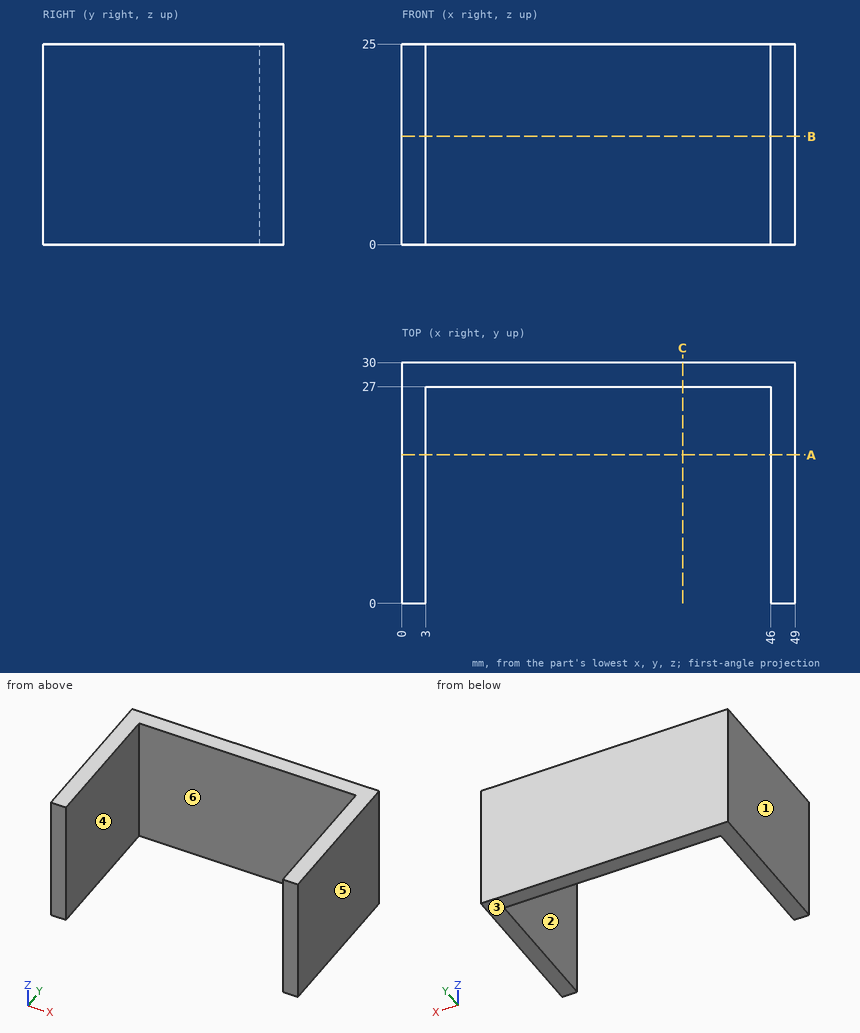
Geometry: see drawing. Coordinates: mm, zero at the bounding-box minimum. A direction names the side the tool comes from. Coordinates: 2 decimals unless noted, no trailing zeros. Loops run counter-clockwise (first coordinate to the right, second up) from the corner with the lowest first, then second, coordinate; pieces in that order, holes last. Notation, with made-up numbers: (18, 14.5) - (47, 14.5) arc R15 cw to (47, 35.5) - close; hole circle Ø10 at (27.25, 26.5). An arc over 180 degrees is marked (long way). Answer in a Markdown table with one row per item.
(1) Set-up query: the marked faces 5 and 6. Return all of +Z, -Z, +X, -X, +Y, -Y with unobstructed straight access to the full face (end or side cutting, diameter ignored); none if empty.
Model answer:
| item | result |
|---|---|
| face 5 | +Z, -Z, +X, +Y, -Y |
| face 6 | +Z, -Z, -Y |
(2) Cut plane C-C on x = 35. Output: boundary loops of the cut face in (y, z), plus the area to 3 significant figures.
Model answer:
| item | result |
|---|---|
| outline | (27, 0) - (30, 0) - (30, 25) - (27, 25) - close |
| area | 75.0 mm² |
(3) Pin query (flat end, axial travel): P1, Ø1, axis at x = 13, z = 9.5, coming from the -Y side. Return the tip coordinate at first contact, or that it passes through.
Model answer:
| item | result |
|---|---|
| P1 | stops at y = 27 |
(4) Material intervals for L1, parallel to X at y = 8.75, z = 16.5; L2, parallel to Y at x = 20, z = 21, sorted ascending. Write a range as from..to.
Model answer:
| item | result |
|---|---|
| L1 | x = 0..3, 46..49 |
| L2 | y = 27..30 |
(5) Cut plane B-B on z = 13.5. Output: boundary loops of the cut face in (x, y), plus the area to 3 significant figures.
Model answer:
| item | result |
|---|---|
| outline | (0, 0) - (3, 0) - (3, 27) - (46, 27) - (46, 0) - (49, 0) - (49, 30) - (0, 30) - close |
| area | 309 mm² |
(6) Mould query, pull axis X, two halves, no side actions, for the marked faces 1, 2, 3 and 4. Classes: pulls with the +X half, pulls with the -X half, needs draft (parallel to the pull), parting line crosses it, or undercut.
Model answer:
| item | result |
|---|---|
| face 1 | pulls with the -X half |
| face 2 | undercut |
| face 3 | needs draft |
| face 4 | undercut |
(7) Cut plane A-A on y = 18.5. Output: boundary loops of the cut face in (x, z).
Model answer:
| item | result |
|---|---|
| outline | (0, 0) - (3, 0) - (3, 25) - (0, 25) - close; (46, 0) - (49, 0) - (49, 25) - (46, 25) - close |
